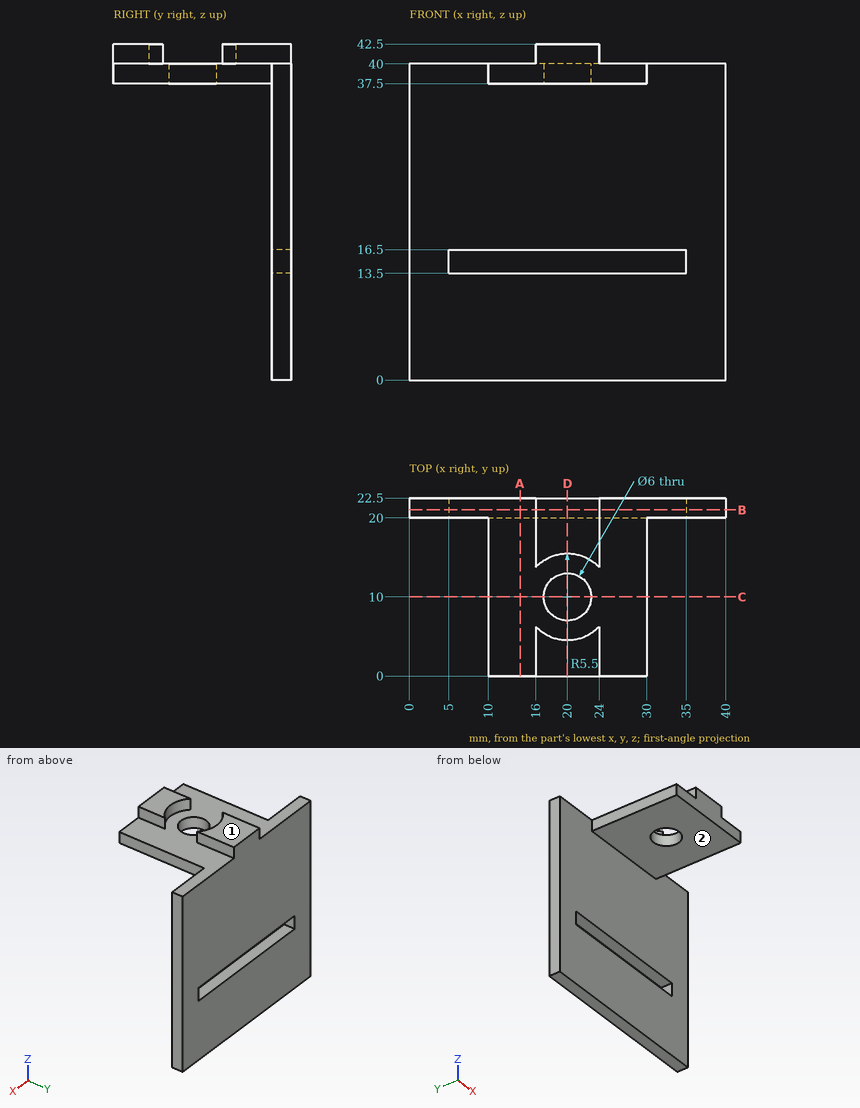
Drawing for the job (mm, zero at the part's lowest x, y, z). A direction names the side the tool comes from. Round coordinates to 2 decimals unless told otherwise and drop trailing zeros. Write each loop counter-clockwise with the first axis right and the second up, starting at its lowest first coordinate (ties: lowest second). Pieces come first, ordered by that corner, then holes.
Item 1: Band-saw the part on D-D on x = 20. Write the cut outline in (y, z).
Filled in:
outline: (0, 37.5) - (7, 37.5) - (7, 40) - (4.5, 40) - (4.5, 42.5) - (0, 42.5) - close; (13, 37.5) - (20, 37.5) - (20, 16.5) - (22.5, 16.5) - (22.5, 42.5) - (15.5, 42.5) - (15.5, 40) - (13, 40) - close; (20, 0) - (22.5, 0) - (22.5, 13.5) - (20, 13.5) - close
Item 2: Band-saw the part on B-B on y = 21. Write the cut outline in (x, z).
Filled in:
outline: (0, 0) - (40, 0) - (40, 40) - (24, 40) - (24, 42.5) - (16, 42.5) - (16, 40) - (0, 40) - close; hole (5, 13.5) - (35, 13.5) - (35, 16.5) - (5, 16.5) - close
Item 3: Band-saw the part on A-A on x = 14. Write the cut outline in (y, z), then the cut area to 4 significant figures.
Filled in:
outline: (0, 37.5) - (20, 37.5) - (20, 16.5) - (22.5, 16.5) - (22.5, 40) - (0, 40) - close; (20, 0) - (22.5, 0) - (22.5, 13.5) - (20, 13.5) - close
area: 142.5 mm2
Item 4: Drill centre lines: L1, parallel to X at y = 10, z = 38.3; L2, parallel to Y at x = 20, z = 39.25; L3, parallel to Y at x = 7.5, z = 11.5. Where is each one in solid material? Low to high.
Filled in:
L1: x = 10 to 17, 23 to 30
L2: y = 0 to 7, 13 to 22.5
L3: y = 20 to 22.5
Item 5: Band-saw the part on C-C on y = 10. Write the cut outline in (x, z), then the cut area to 3 significant figures.
Filled in:
outline: (10, 37.5) - (17, 37.5) - (17, 40) - (10, 40) - close; (23, 37.5) - (30, 37.5) - (30, 40) - (23, 40) - close
area: 35.0 mm2
Item 6: Drop flat-ended pins along their axis: pin 1 Ø2 at (x, y) = (14.5, 22) entering from +Z; pin 2 Ø0.8 at (y, z) = (4, 41.5) entering from -X; pin 3 Ø2 at (y, z) = (12.5, 38.5) entering from +X; pin 4 Ø2 at (x, y) = (8.5, 14) entering from +Z. Give the stop position or say it passes through.
Filled in:
pin 1: stops at z = 40
pin 2: stops at x = 16
pin 3: stops at x = 30
pin 4: passes through
Item 7: Tool access for the marked faces 1 and 2: list every direction of +Z, -Z, +X, -X, +Y, -Y with a clear straight run to the whole face (end or side of a thin tool).
Filled in:
face 1: +Z, +X, -X, +Y, -Y
face 2: -Z, +X, -X, -Y
